from build123d import *

# Parameters (mm, degrees)
EXTRUDE_1_DEPTH = 1
CHAMFER_1_SIZE  = 0.5
SKETCH_2_R      = 0.55
EXTRUDE_2_DEPTH = 1.9


with BuildPart() as part:
    # 草图1 → 凸台-拉伸1 (new body)
    with BuildSketch(Plane.XY):
        with BuildLine():
            Line((-7.237622799, 4.594383921), (-12.737622799, 4.594383921))
            ThreePointArc((-12.737622799, 4.594383921), (-13.091176189, 4.74083053), (-13.237622799, 5.094383921))
            Line((-13.237622799, 5.094383921), (-13.237622799, 9.594383921))
            ThreePointArc((-13.237622799, 9.594383921), (-13.091176189, 9.947937312), (-12.737622799, 10.094383921))
            Line((-12.737622799, 10.094383921), (-7.237622799, 10.094383921))
            ThreePointArc((-7.237622799, 10.094383921), (-6.884069408, 9.947937312), (-6.737622799, 9.594383921))
            Line((-6.737622799, 9.594383921), (-6.737622799, 5.094383921))
            ThreePointArc((-6.737622799, 5.094383921), (-6.884069408, 4.74083053), (-7.237622799, 4.594383921))
        make_face()
    extrude(amount=EXTRUDE_1_DEPTH)

    # 倒角1
    chamfer_1_edges = [part.edges().sort_by_distance(p)[0] for p in [
        (-13.091176189, 9.947937312, 1),
        (-13.237622799, 7.344383921, 1),
        (-13.091176189, 4.74083053, 1),
        (-9.987622799, 4.594383921, 1),
        (-6.884069408, 4.74083053, 1),
        (-6.737622799, 7.344383921, 1),
        (-6.884069408, 9.947937312, 1),
        (-9.987622799, 10.094383921, 1),
    ]]
    chamfer(chamfer_1_edges, length=CHAMFER_1_SIZE - 0.0001)  # a hair under: the kernel refuses the full size

    # 草图2 → 凸台-拉伸2 (add)
    with BuildSketch(Plane(origin=(0, 0, 0), x_dir=(-1, 0, 0), z_dir=(0, 0, -1))):
        with Locations(Location((11.737622799, 7.344383921, 0), (0, 0, 180))):
            Circle(SKETCH_2_R)
        with Locations(Location((8.237622799, 7.344383921, 0), (0, 0, 180))):
            Circle(SKETCH_2_R)
    extrude(amount=EXTRUDE_2_DEPTH)


solid = part.part
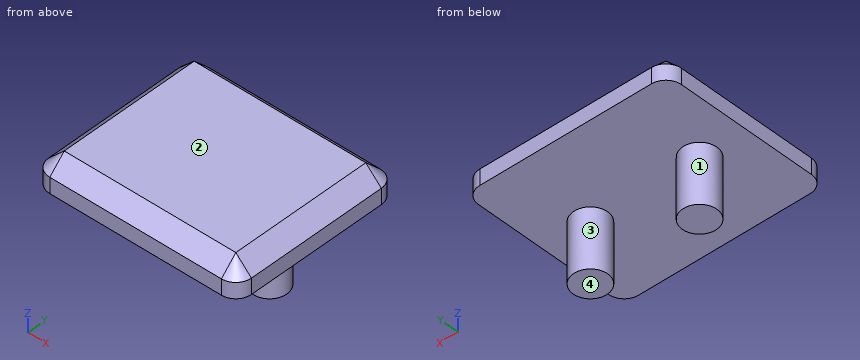
Geometry check sheet. Reference: the model listing, model coordinates, mm. Face numbers are marked on the shaded views. A direction names the side the tool comes from. Give positions to 0.01 mm unless a question says otherwise; leave off trailing zeros. Order: outer loops, then holes, each group sorted by start corner. A loop starts at its lowest first (then second) coordinate and runs counter-clockwise, first axis right, second up. Notation, with made-up numbers: M 40.25,38.25 L 97.25,38.25 A11 cw 97.25,43.25 Z; hole C 8,-24.75 d3. An arc over 180 degrees is marked long. Use a Markdown table: item, result.
Item 1: Section check D-D (z = -1.65). Record the cut outline in (x, y).
Answers follow:
| item | result |
|---|---|
| outline | C -11.74,7.34 d1.1; C -8.24,7.34 d1.1 |
Item 2: Section check B-B (z = 0.85). Record the cut outline in (x, y), and give its area (3 significant figures).
Answers follow:
| item | result |
|---|---|
| outline | M -12.89,5.09 A0.15 ccw -12.74,4.94 L -7.24,4.94 A0.15 ccw -7.09,5.09 L -7.09,9.59 A0.15 ccw -7.24,9.74 L -12.74,9.74 A0.15 ccw -12.89,9.59 Z |
| area | 27.8 mm2 |
Item 3: Depth check by flat-ended pin: P1, Ø1, axis at x = -8.5, z = -1.5, coming from the -Y side. Enter the tip coordinate at first touch or a pass-through.
Answers follow:
| item | result |
|---|---|
| P1 | stops at y = 6.79 |
Item 4: Section check A-A (x = -10). Record the cut outline in (y, z).
Answers follow:
| item | result |
|---|---|
| outline | M 4.59,0 L 10.09,0 L 10.09,0.5 L 9.59,1 L 5.09,1 L 4.59,0.5 Z |
Item 5: Draft check along X on the marked faces 3 and 4. Enter one of: +X half, -X half, draft (parallel to the pull), parting line (faces both ways), or undercut.
Answers follow:
| item | result |
|---|---|
| face 3 | undercut |
| face 4 | draft |
Item 6: Tool access check on the marked faces 1 and 2. Record the directions out of +Z, -Z, +X, -X, +Y, -Y that give a thin tool (end or side, any length) a straight path to the whole face; none if there is none.
Answers follow:
| item | result |
|---|---|
| face 1 | -Z |
| face 2 | +Z, +X, -X, +Y, -Y |
Item 7: Material ranges on line 1 along Z through (x, y) = (-8.25, 5.6); line 2 along X through (y, z) = (7, -0.75); line 3 along X through (y, z) = (7.55, -0.95), recorded low to high.
Answers follow:
| item | result |
|---|---|
| line 1 | z = 0 to 1 |
| line 2 | x = -12.17 to -11.31, -8.67 to -7.81 |
| line 3 | x = -12.25 to -11.23, -8.75 to -7.73 |
Item 8: Section check C-C (y = 8.2). Record the cut outline in (x, z), and give its area (3 significant figures).
Answers follow:
| item | result |
|---|---|
| outline | M -13.24,0 L -6.74,0 L -6.74,0.5 L -7.24,1 L -12.74,1 L -13.24,0.5 Z |
| area | 6.25 mm2 |
